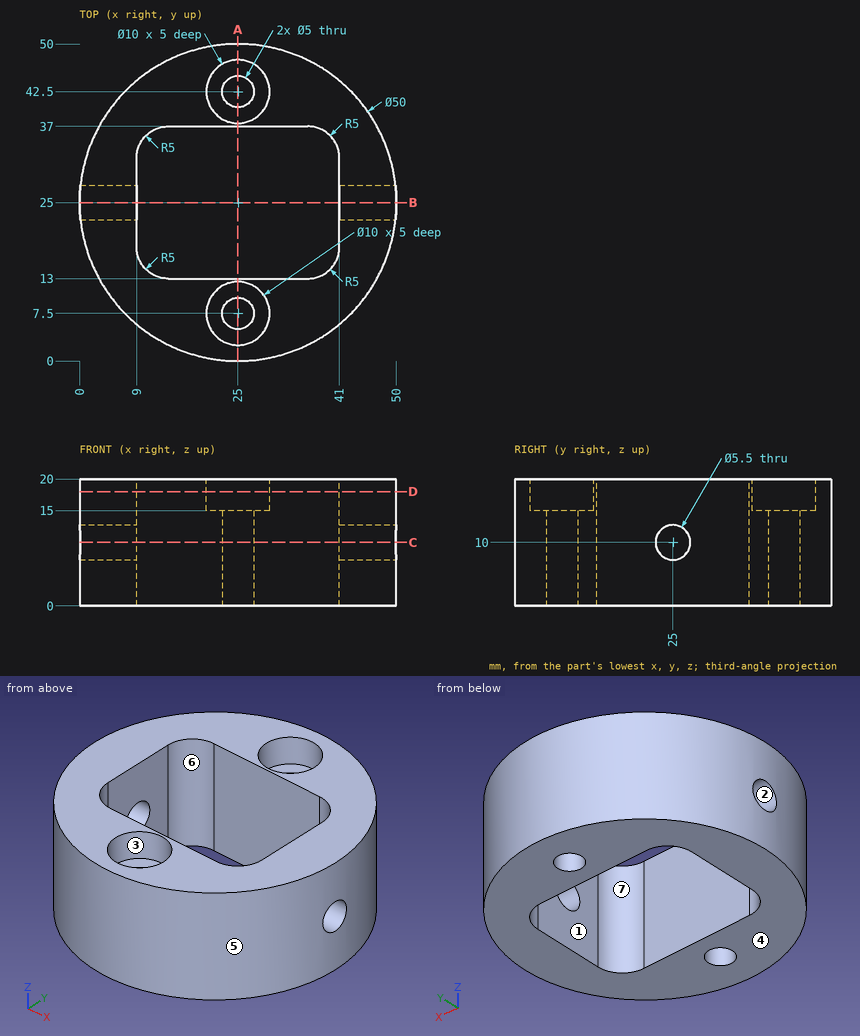
For this review, use the dimensioned drawing (mm, ordinates from the lowest corner) and the shaded views. A direction names the side the tool comes from. Round coordinates to 2 decimals unless told otherwise and drop trailing zeros. Order: outer loops, then holes, each group sorted by start corner. A loop starts at its lowest first (then second) coordinate and runs counter-clockwise, first axis right, second up. Notation, with made-up numbers: M 69,-25 L 108,-25 A15 ccw 108,-12 Z; hole C -38.5,5 d10. An arc over 180 degrees is marked long. Use a Markdown table: item, result.
1) Consider section C-C (z = 10). Write out the cut boundary in (x, y), then the cut area to 3 significant figures.
Report:
| item | result |
|---|---|
| outline | M 0.15,22.25 A25 ccw 49.85,22.25 L 41,22.25 L 41,18 A5 cw 36,13 L 14,13 A5 cw 9,18 L 9,22.25 Z; M 0.15,27.75 L 9,27.75 L 9,32 A5 cw 14,37 L 36,37 A5 cw 41,32 L 41,27.75 L 49.85,27.75 A25 ccw Z; hole C 25,7.5 d5; hole C 25,42.5 d5 |
| area | 1,080 mm^2 |
2) Wall thickness on line 1 along Y through (x, z) = (25, 10.25); line 2 along Z through (x, y) = (48, 25); line 3 along Y through (x, z) = (17.5, 17.5): over which ranges is each line inside the solid? List them lowest first. Write a range as [from, to].
Report:
| item | result |
|---|---|
| line 1 | [0, 5], [10, 13], [37, 40], [45, 50] |
| line 2 | [0, 7.25], [12.75, 20] |
| line 3 | [1.15, 13], [37, 48.85] |
3) Consider section B-B (y = 25). Write out the cut boundary in (x, z), then the cut area to 3 significant figures.
Report:
| item | result |
|---|---|
| outline | M 0,0 L 9,0 L 9,7.25 L 0,7.25 Z; M 0,12.75 L 9,12.75 L 9,20 L 0,20 Z; M 41,0 L 50,0 L 50,7.25 L 41,7.25 Z; M 41,12.75 L 50,12.75 L 50,20 L 41,20 Z |
| area | 261 mm^2 |
4) Consider section D-D (z = 18). Write out the cut boundary in (x, y).
Report:
| item | result |
|---|---|
| outline | C 25,25 d50; hole M 9,18 A5 ccw 14,13 L 36,13 A5 ccw 41,18 L 41,32 A5 ccw 36,37 L 14,37 A5 ccw 9,32 Z; hole C 25,7.5 d10; hole C 25,42.5 d10 |
5) Draft analysis for pull direction Y (two halves, no side actions). For the marked faces 4, 5, 6 and 7, state which applies: released by +Y, released by -Y, zero draft, split by the parting line, or undercut.
Report:
| item | result |
|---|---|
| face 4 | zero draft |
| face 5 | split by the parting line |
| face 6 | undercut |
| face 7 | undercut |
6) Tool access review of the marked faces 1, 2 and 3: name each direction out of +Z, -Z, +X, -X, +Y, -Y from which nothing blocks a thin tool from reaching the whole face with its end or side.
Report:
| item | result |
|---|---|
| face 1 | +Z, -Z |
| face 2 | +X, -X |
| face 3 | +Z |
7) Consider section A-A (x = 25). Write out the cut boundary in (y, z), then the cut area to 3 significant figures.
Report:
| item | result |
|---|---|
| outline | M 0,0 L 5,0 L 5,15 L 2.5,15 L 2.5,20 L 0,20 Z; M 10,0 L 13,0 L 13,20 L 12.5,20 L 12.5,15 L 10,15 Z; M 37,0 L 40,0 L 40,15 L 37.5,15 L 37.5,20 L 37,20 Z; M 45,0 L 50,0 L 50,20 L 47.5,20 L 47.5,15 L 45,15 Z |
| area | 270 mm^2 |
8) Insertion check: pin 1 (1 mm diameter, centred on y = 21, z = 4.5, fed in from +X); pin 2 (10 mm diameter, centred on x = 27, z = 12, fed in from -Y); pin 3 (12 mm diameter, centred on x = 40.5, z = 15, fed in from +Y). Each pin has a flat end and moves straight along its axis. Give the tip position at first contact, or say it passes through.
Report:
| item | result |
|---|---|
| pin 1 | x = 49.75 |
| pin 2 | y = 0 |
| pin 3 | y = 48.12 |
